Design review of the part built by this model. Coordinates are the model's own, in mm. A direction names the side the tool comes from. Coordinates: 2 decimals unless noted, no trailing zeros. Loops run counter-clockwise (first coordinate to the right, second up) from the corner with the lowest first, then second, coordinate; pieces in that order, holes last. Notation, with made-up numbers: (-23, 20.5) -> (10, 20.5) arc R18 ccw to (10, 51.5) -> close; hole circle Ø8 at (49.5, 81). An arc over 180 degrees is marked (long way). Answer in a Markdown table with one row per item.
```python
from build123d import *

# Parameters (mm, degrees)
SCHIZZO1_W                   = 110.21
SCHIZZO1_H                   = 110.21
ESTRUSIONE_ESTRUSIONE1_DEPTH = 10
RACCORDO1_R                  = 10
SCHIZZO6_W                   = 25
SCHIZZO6_H                   = 25
ESTRUSIONE_ESTRUSIONE2_DEPTH = 25
RACCORDO2_R                  = 5
SCHIZZO8_W                   = 47.3
SCHIZZO8_H                   = 47.3
SCHIZZO8_W_2                 = 42.3
SCHIZZO8_H_2                 = 42.3
ESTRUSIONE_ESTRUSIONE4_DEPTH = 30
SCHIZZO16_W                  = 4
SCHIZZO16_H                  = 10
TAGLIO_ESTRUSIONE11_DEPTH    = 10
SCHIZZO20_R                  = 7.8
TAGLIO_ESTRUSIONE12_DEPTH    = 25
RACCORDO11_R                 = 5
RACCORDO12_R                 = 5
RACCORDO13_R                 = 5
SCHIZZO10_W                  = 95.163374128
SCHIZZO10_H                  = 10
ESTRUSIONE_ESTRUSIONE5_DEPTH = 30
SCHIZZO21_R                  = 4.15
TAGLIO_ESTRUSIONE13_DEPTH    = 17
RACCORDO15_R                 = 5
RACCORDO16_R                 = 2
RACCORDO15_OF_SPECCHIA20_R   = 5
RACCORDO16_OF_SPECCHIA20_R   = 2
ESTRUSIONE_ESTRUSIONE7_REACH = 106.11
TAGLIO_ESTRUSIONE16_DEPTH    = 8.05
RACCORDO18_R                 = 1
TAGLIO_ESTRUSIONE14_DEPTH    = 17


with BuildPart() as part:
    # Schizzo1 → Estrusione-Estrusione1 (new body)
    with BuildSketch(Plane.XY):
        Rectangle(SCHIZZO1_W, SCHIZZO1_H)
    extrude(amount=ESTRUSIONE_ESTRUSIONE1_DEPTH)

    # Raccordo1
    raccordo1_edges = [part.edges().sort_by_distance(p)[0] for p in [
        (55.105, -55.105, 5),
        (-55.105, -55.105, 5),
        (-55.105, 55.105, 5),
        (55.105, 55.105, 5),
    ]]
    fillet(raccordo1_edges, radius=RACCORDO1_R)

    # Schizzo6 → Estrusione-Estrusione2 (add)
    with BuildSketch(Plane(origin=(0, 0, 0), x_dir=(-1, 0, 0), z_dir=(0, 0, -1))):
        with Locations((-32.605, 32.605)):
            Rectangle(SCHIZZO6_W, SCHIZZO6_H)
        with Locations((-32.605, -32.605)):
            Rectangle(SCHIZZO6_W, SCHIZZO6_H)
    estrusione_estrusione2 = extrude(amount=ESTRUSIONE_ESTRUSIONE2_DEPTH)

    # Raccordo2
    raccordo2_edges = [part.edges().sort_by_distance(p)[0] for p in [
        (32.605, 20.105, -25),
        (32.605, 45.105, -25),
    ]]
    fillet(raccordo2_edges, radius=RACCORDO2_R)

    # Schizzo8 → Estrusione-Estrusione4 (add)
    with BuildSketch(Plane.XY.offset(10)):
        Rectangle(SCHIZZO8_W, SCHIZZO8_H)
        Rectangle(SCHIZZO8_W_2, SCHIZZO8_H_2, mode=Mode.SUBTRACT)
    extrude(amount=ESTRUSIONE_ESTRUSIONE4_DEPTH)

    # Schizzo16 → Taglio-Estrusione11 (cut)
    with BuildSketch(Plane(origin=(0, 0, 0), x_dir=(-1, 0, 0), z_dir=(0, 0, -1))):
        with Locations((-48.105, 0)):
            Rectangle(SCHIZZO16_W, SCHIZZO16_H)
        with Locations((48.105, 0)):
            Rectangle(SCHIZZO16_W, SCHIZZO16_H)
    extrude(amount=-TAGLIO_ESTRUSIONE11_DEPTH, mode=Mode.SUBTRACT)

    # Schizzo20 → Taglio-Estrusione12 (cut)
    with BuildSketch(Plane(origin=(45.105, 0, 0), x_dir=(0, 0, -1), z_dir=(1, 0, 0))):
        with Locations((13.030698379, 33.188614524)):
            Circle(SCHIZZO20_R)
        with Locations(Location((13.030698379, -33.188614524, 0), (0, 0, 180))):
            Circle(SCHIZZO20_R)
    taglio_estrusione12 = extrude(amount=-TAGLIO_ESTRUSIONE12_DEPTH, mode=Mode.SUBTRACT)

    # Raccordo11
    raccordo11_edges = [part.edges().sort_by_distance(p)[0] for p in [
        (32.605, -20.105, -25),
    ]]
    fillet(raccordo11_edges, radius=RACCORDO11_R)

    # Raccordo12
    raccordo12_edges = [part.edges().sort_by_distance(p)[0] for p in [
        (32.605, -45.105, -25),
    ]]
    fillet(raccordo12_edges, radius=RACCORDO12_R)

    # Specchia17: Estrusione-Estrusione2 across plane
    add(estrusione_estrusione2.mirror(Plane(origin=(0, 0, 0), x_dir=(0, 0, 1), z_dir=(1, 0, 0))))

    # Specchia19: Taglio-Estrusione12 across plane
    add(taglio_estrusione12.mirror(Plane(origin=(0, 0, 0), x_dir=(0, 0, 1), z_dir=(1, 0, 0))), mode=Mode.SUBTRACT)

    # Raccordo13
    raccordo13_edges = [part.edges().sort_by_distance(p)[0] for p in [
        (-32.605, 45.105, -25),
        (-32.605, 20.105, -25),
        (-32.605, -45.105, -25),
        (-32.605, -20.105, -25),
    ]]
    fillet(raccordo13_edges, radius=RACCORDO13_R)

    # Schizzo10 → Estrusione-Estrusione5 (add)
    with BuildSketch(Plane.XY.offset(10)):
        with Locations((0, -36.820977582)):
            Rectangle(SCHIZZO10_W, SCHIZZO10_H)
    estrusione_estrusione5 = extrude(amount=ESTRUSIONE_ESTRUSIONE5_DEPTH)

    # Schizzo21 → Taglio-Estrusione13 (cut)
    with BuildSketch(Plane.XZ.offset(41.820977582)):
        with Locations(Location((-38.020045692, 31.433841087, 0), (0, 0, 270))):
            Circle(SCHIZZO21_R)
        with Locations(Location((38.020045692, 31.433841087, 0), (0, 0, 90))):
            Circle(SCHIZZO21_R)
        Polygon((-28.203808042, 40), (-23.137362803, 28.426939363), (23.137362803, 28.426939363), (28.203808042, 40), align=None)
    taglio_estrusione13 = extrude(amount=-TAGLIO_ESTRUSIONE13_DEPTH, mode=Mode.SUBTRACT)

    # Raccordo15
    raccordo15_edges = [part.edges().sort_by_distance(p)[0] for p in [
        (47.581687064, -36.820977582, 40),
        (-47.581687064, -36.820977582, 40),
        (-28.203808042, -36.820977582, 40),
        (28.203808042, -36.820977582, 40),
    ]]
    fillet(raccordo15_edges, radius=RACCORDO15_R)

    # Raccordo16
    raccordo16_edges = [part.edges().sort_by_distance(p)[0] for p in [
        (-47.581687064, -36.820977582, 10),
        (0, -41.820977582, 10),
        (0, -31.820977582, 10),
        (47.581687064, -36.820977582, 10),
    ]]
    fillet(raccordo16_edges, radius=RACCORDO16_R)

    # Specchia20: Estrusione-Estrusione5, Taglio-Estrusione13 across plane
    add(estrusione_estrusione5.mirror(Plane.ZX))
    add(taglio_estrusione13.mirror(Plane.ZX), mode=Mode.SUBTRACT)

    # Raccordo15 of Specchia20
    raccordo15_of_specchia20_edges = [part.edges().sort_by_distance(p)[0] for p in [
        (47.581687064, 36.820977582, 40),
        (-47.581687064, 36.820977582, 40),
        (-28.203808042, 36.820977582, 40),
        (28.203808042, 36.820977582, 40),
    ]]
    fillet(raccordo15_of_specchia20_edges, radius=RACCORDO15_OF_SPECCHIA20_R)

    # Raccordo16 of Specchia20
    raccordo16_of_specchia20_edges = [part.edges().sort_by_distance(p)[0] for p in [
        (-47.581687064, 36.820977582, 10),
        (0, 41.820977582, 10),
        (0, 31.820977582, 10),
        (47.581687064, 36.820977582, 10),
    ]]
    fillet(raccordo16_of_specchia20_edges, radius=RACCORDO16_OF_SPECCHIA20_R)

    # Estrusione-Estrusione7: up to this face of the body (flat: up to its plane)
    estrusione_estrusione7_end = Plane(part.part.faces().sort_by_distance((23.65, 0, 25))[0])
    # Schizzo29 → Estrusione-Estrusione7 (add, up to the picked face)
    with BuildSketch(Plane.ZY.offset(23.65), mode=Mode.PRIVATE) as estrusione_estrusione7_sk1:
        Polygon((40, 23.65), (28.426939363, 31.820977582), (10, 31.820977582), (10, 23.65), align=None)
    estrusione_estrusione7_tool1 = split(extrude(estrusione_estrusione7_sk1.sketch, amount=-ESTRUSIONE_ESTRUSIONE7_REACH, mode=Mode.PRIVATE), bisect_by=estrusione_estrusione7_end, keep=Keep.BOTH, mode=Mode.PRIVATE)
    estrusione_estrusione7 = estrusione_estrusione7_tool1.solids().sort_by(Axis((-23.65, 27.410039, 22.337212), (1, 0, 0)))[0]
    add(estrusione_estrusione7)

    # Specchia22: Estrusione-Estrusione7 across plane
    add(estrusione_estrusione7.mirror(Plane.ZX))

    # Schizzo30 → Taglio-Estrusione16 (cut)
    with BuildSketch(Plane(origin=(23.65, 0, 0), x_dir=(0, 0, -1), z_dir=(1, 0, 0))):
        Polygon((-16, -4), (-10, -5.843863655), (-10, -4), (-10, 4), (-10, 5.843863655), (-16, 4), align=None)
    extrude(amount=-TAGLIO_ESTRUSIONE16_DEPTH, mode=Mode.SUBTRACT)

    # Raccordo18
    raccordo18_edges = [part.edges().sort_by_distance(p)[0] for p in [
        (22.4, -5.843863655, 10),
        (22.4, -4, 16),
        (22.4, 4, 16),
        (22.4, 5.843863655, 10),
    ]]
    fillet(raccordo18_edges, radius=RACCORDO18_R)

    # Schizzo28 → Taglio-Estrusione14 (cut)
    with BuildSketch(Plane.ZY.offset(-21.15)):
        with BuildLine():
            Line((10, 4.773633228), (10, -4.589423386))
            ThreePointArc((10, -4.589423386), (14.681528307, 0.092104921), (10, 4.773633228))
        make_face()
    extrude(amount=-TAGLIO_ESTRUSIONE14_DEPTH, mode=Mode.SUBTRACT)


solid = part.part
```
(1) Take a section at A-A on z = -2. Give the boundary of the cut face in (x, y) (3 decimals), and give its area (3 significant figures).
Evaluation:
| item | result |
|---|---|
| outline | (-45.105, -45.105) -> (-20.105, -45.105) -> (-20.105, -20.105) -> (-45.105, -20.105) -> close; (-45.105, 20.105) -> (-20.105, 20.105) -> (-20.105, 45.105) -> (-45.105, 45.105) -> close; (20.105, -45.105) -> (45.105, -45.105) -> (45.105, -20.105) -> (20.105, -20.105) -> close; (20.105, 20.105) -> (45.105, 20.105) -> (45.105, 45.105) -> (20.105, 45.105) -> close |
| area | 2,500 mm² |
(2) Draft analysis for pull direction Y (two halves, no side actions). For faces 6 (the flat face through (33, -45.105, -10)), 7 (the flat face through (33, 20.105, -10)), 8 (the flat face through (-1, 1, 0)), 9 (the flat face through (-45.105, -27, -7)), state which applies: pulls with the +Y half, pulls with the -Y half, needs draft (parallel to the pull), parting line crosses it, or undercut.
Evaluation:
| item | result |
|---|---|
| face 6 | pulls with the -Y half |
| face 7 | undercut |
| face 8 | undercut |
| face 9 | needs draft |
(3) To check wall thickness, follow probe 1 along Y at (x, z) = (-29, -3.5) (3 decimals); probe 2 along Y at (x, z) = (47, 36); probe 3 along Y at (x, z) = (-38, -16.5) (3 decimals). State the ranges of each line that lie inside material, in increasing order.
Evaluation:
| item | result |
|---|---|
| probe 1 | y = -45.105 to -20.105, 20.105 to 45.105 |
| probe 2 | y = -41.82 to -31.82, 31.82 to 41.82 |
| probe 3 | y = -45.105 to -40.175, -26.203 to -20.105, 20.105 to 26.203, 40.175 to 45.105 |
(4) Take a section at B-B on y = 10.5. Give the boundary of the cut face in (x, z) (3 decimals).
Evaluation:
| item | result |
|---|---|
| outline | (-55.105, 0) -> (55.105, 0) -> (55.105, 10) -> (23.65, 10) -> (23.65, 40) -> (21.15, 40) -> (21.15, 10) -> (-21.15, 10) -> (-21.15, 40) -> (-23.65, 40) -> (-23.65, 10) -> (-55.105, 10) -> close |
(5) Tool access review of faces 1 (the flat face through (33, -20.105, -10)), 2 (the flat face through (45.105, -27, -7)), 3 (the flat face through (-1, 41.821, 23)), 4 (the flat face through (0, -37, 28.427)), 5 (the flat face through (-33, 45.105, -10)): name each direction out of +Z, -Z, +X, -X, +Y, -Y from which nothing blocks a thin tool from reaching the whole face with its end or side.
Evaluation:
| item | result |
|---|---|
| face 1 | -Z, +X, -X |
| face 2 | -Z, +X, +Y, -Y |
| face 3 | +Z, +X, -X, +Y |
| face 4 | +Z, -Y |
| face 5 | -Z, +X, -X, +Y |
(6) Take a section at D-D on x = -29.5. Count the separate pieces of the cut face and the enclosed holes in it, and give its area (3 significant figures).
Evaluation:
| item | result |
|---|---|
| separate pieces | 1 |
| enclosed holes | 2 |
| area | 2,540 mm² |
(7) For pin 1 (10 mm diameter, centred on x = -35, z = -6.5, fed in from -Y) (3 decimals); pin 2 (10 mm diameter, centred on x = 15, y = 6, fed in from +Z); pin 3 (1.5 mm diameter, centred on x = -31.5, z = 23.5, fed in from -Y), all flat-tipped, find the tip position at first contact; note any pin that passes through.
Evaluation:
| item | result |
|---|---|
| pin 1 | stops at y = -45.105 |
| pin 2 | stops at z = 10 |
| pin 3 | stops at y = -41.82 |
(8) Take a section at C-C on x = 4. Give the boundary of the cut face in (y, z) (3 decimals), and give its area (3 significant figures).
Evaluation:
| item | result |
|---|---|
| outline | (-55.105, 0) -> (55.105, 0) -> (55.105, 10) -> (43.821, 10) arc R2 cw to (41.821, 12) -> (41.821, 28.427) -> (31.821, 28.427) -> (23.65, 40) -> (21.15, 40) -> (21.15, 10) -> (-21.15, 10) -> (-21.15, 40) -> (-23.65, 40) -> (-31.821, 28.427) -> (-41.821, 28.427) -> (-41.821, 12) arc R2 cw to (-43.821, 10) -> (-55.105, 10) -> close |
| area | 2,020 mm² |
